Here's how the part is built. I have some questions about the finished solid (model axes, mm). A direction names the side the tool comes from. Coordinates: 2 decimals unless noted, no trailing zeros. Loops run counter-clockwise (first coordinate to the right, second up) from the corner with the lowest first, then second, coordinate; pieces in that order, holes last. Notation, with made-up numbers: (47.5, 62) -> (97.5, 62) arc R19 ccw to (97.5, 94) -> close; hole circle Ø2 at (-37.75, 61.5). An arc over 180 degrees is marked (long way). Answer as a JSON object with one key per item and string values. Group by question number.
1) I want a section at A-A (x = -33.75). Write out the boundary of the cut face in (y, z).
2) Which directions (+Z, -Z, +X, -X, +Y, -Y) give clear straight access to the entire face, cutting with the end or side of a thin tool? Please do faces 1 (the flat face through (-31, -1.58, 25)), 2 (the flat face through (-28, -4, 25.12)), 3 (the flat face through (-26.613, -4, 24)), 4 (the flat face through (-34, -4, 26.64)).
3) If we mould it in two halves opening along Z, with no side actions, what happens to faces 5 (the cylindrical face through (-27.419, -4.134, 30.267)), 6 (the flat face through (-31, -6.4, 25)), 7 (the flat face through (-34, -4, 31.55)), 8 (the flat face through (-31, -4, 31.71))? For each: +Z half, -Z half, draft (parallel to the pull), parting line (faces both ways), or undercut.
4) I want a section at C-C (x = -27.5). Write out the boundary of the cut face in (y, z) (3 decimals).
5) I want a section at B-B (z = 25.25). Write out the boundary of the cut face in (x, y).
6) I need wall thicknesses on probe 1 along Z at (x, y) = (-28, -4); probe 2 along Y at (x, z) = (-31.5, 30.25); probe 3 along Y at (x, z) = (-31.75, 24.75). Which ranges of each line are inside material? Lowest first, please. Write a range as [from, to].
7) I'm going to push flat-ended pins straight in: pin 1 (1.7 mm diameter, centred on y = -5, z = 24, fed in from +X); pin 2 (1.8 mm diameter, centred on y = -3.935, z = 28.755, fed in from -X); pin 3 (1.4 mm diameter, centred on y = -3.5, z = 29.5, fed in from -X). Where does each tip first touch, or does it pass through?
```python
from build123d import *

# Parameters (mm, degrees)
F1_DEPTH  = 7.87
F2_W      = 4.88
F2_H      = 4.91
F3_DEPTH  = 5.81
F4_W      = 4.39
F4_H      = 0.95
F5_DEPTH  = 1.95
F6_W      = 4.74
F6_H      = 4.82
F7_DEPTH  = 8.11
F8_R      = 2.475
F9_DEPTH  = 1.73
F10_R     = 1.525
F11_DEPTH = 25
F12_R     = 2.405
F13_DEPTH = 1.73
F14_R     = 0.217279


with BuildPart() as f1:
    # F0 (on Front) → F1 (new body)
    with BuildSketch(Plane.XZ):
        Polygon((-28.082503, 33.1), (-34.462503, 33.1), (-34.462503, 23.6), (-26.612503, 23.6), (-26.612503, 25.12), (-28.082503, 25.12), align=None)
    extrude(amount=F1_DEPTH)

    # F2 (on face) → F3 (cut)
    with BuildSketch(Plane(origin=(-34.462503, 0, 0), x_dir=(0, -1, 0), z_dir=(-1, 0, 0))):
        with Locations((3.98, 29.095)):
            Rectangle(F2_W, F2_H)
    extrude(amount=-F3_DEPTH, mode=Mode.SUBTRACT)

    # F4 (on face) → F5 (cut)
    with BuildSketch(Plane.YZ.offset(-28.082503)):
        with Locations((-3.815, 25.595)):
            Rectangle(F4_W, F4_H)
    extrude(amount=-F5_DEPTH, mode=Mode.SUBTRACT)

    # F6 (on face) → F7 (cut)
    with BuildSketch(Plane(origin=(0, 0, 23.6), x_dir=(1, 0, 0), z_dir=(0, 0, -1))):
        with Locations((-30.885357, 3.99)):
            Rectangle(F6_W, F6_H)
    extrude(amount=-F7_DEPTH, mode=Mode.SUBTRACT)

    # F8 (on face) → F9 (join)
    with BuildSketch(Plane.YZ.offset(-28.082503)):
        with Locations((-3.935, 28.755)):
            Circle(F8_R)
    extrude(amount=F9_DEPTH)

    # F10 (on face) → F11 (cut)
    with BuildSketch(Plane.YZ.offset(-26.352503)):
        with Locations((-3.935, 28.755)):
            Circle(F10_R)
    extrude(amount=-F11_DEPTH, mode=Mode.SUBTRACT)

    # F12 (on face) → F13 (join)
    with BuildSketch(Plane.XY.offset(33.1)):
        with Locations((-30.486484, -4.005)):
            Circle(F12_R)
        with BuildLine():
            Line((-28.082503, -4.075), (-28.082503, -3.935))
            ThreePointArc((-28.082503, -3.935), (-32.891484, -4.005), (-28.082503, -4.075))
        make_face()
    extrude(amount=F13_DEPTH)

    # F14
    f14_edges = [f1.edges().sort_by_distance(p)[0] for p in [
        (-32.891484, -4.005, 34.83),
    ]]
    fillet(f14_edges, radius=F14_R)


solid = f1.part
```
Determined:
{
 "1": {"outline": "(-7.87, 23.6) -> (0, 23.6) -> (0, 33.1) -> (-7.87, 33.1) -> close; hole (-6.42, 26.64) -> (-1.54, 26.64) -> (-1.54, 31.55) -> (-6.42, 31.55) -> close"},
 "2": {"face 1": "-Z", "face 2": "+X", "face 3": "-Z, +X, +Y, -Y", "face 4": "-X"},
 "3": {"face 5": "undercut", "face 6": "draft", "face 7": "undercut", "face 8": "-Z half"},
 "4": {"outline": "(-7.87, 23.6) -> (0, 23.6) -> (0, 25.12) -> (-7.87, 25.12) -> close; circle Ø4.95 at (-3.935, 28.755); hole circle Ø3.05 at (-3.935, 28.755)"},
 "5": {"outline": "(-34.46, -7.87) -> (-28.08, -7.87) -> (-28.08, -6.01) -> (-28.52, -6.01) -> (-28.52, -6.4) -> (-33.26, -6.4) -> (-33.26, -1.58) -> (-28.52, -1.58) -> (-28.52, -1.62) -> (-28.08, -1.62) -> (-28.08, 0) -> (-34.46, 0) -> close"},
 "6": {"probe 1": "[23.6, 25.12], [26.28, 27.23], [30.28, 31.23]", "probe 2": "[-7.87, -6.42], [-1.54, 0]", "probe 3": "[-7.87, -6.4], [-1.58, 0]"},
 "7": {"pin 1": "x = -26.61", "pin 2": "through", "pin 3": "x = -28.52"}
}
